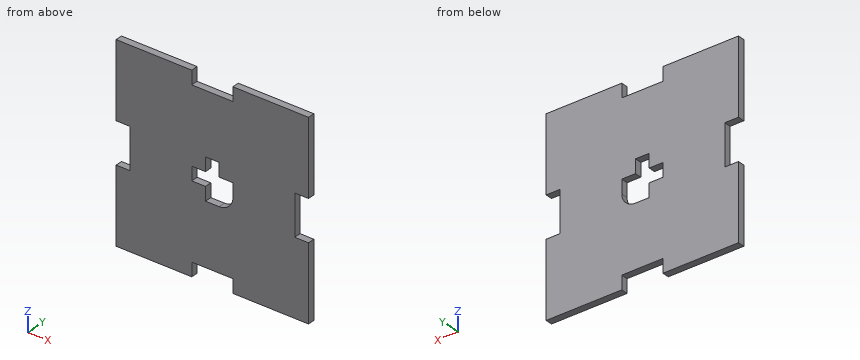
```python
from build123d import *

# Parameters (mm, degrees)
SKETCH1_W           = 88.9
SKETCH1_H           = 88.9
BOSS_EXTRUDE1_DEPTH = 3.175
CUT_EXTRUDE3_DEPTH  = 3.175
SKETCH4_W           = 19.05
SKETCH4_H           = 6.35
SKETCH4_W_2         = 6.35
SKETCH4_H_2         = 19.05
CUT_EXTRUDE2_DEPTH  = 3.175
SKETCH7_W           = 6.35
SKETCH7_H           = 6.35
CUT_EXTRUDE4_DEPTH  = 126.763669734
FILLET1_R           = 6.35


with BuildPart() as part:
    # Sketch1 → Boss-Extrude1 (new body)
    with BuildSketch(Plane(origin=(0, 0, 0), x_dir=(1, 0, 0), z_dir=(0, 1, 0))):
        with Locations((44.45, 44.45)):
            Rectangle(SKETCH1_W, SKETCH1_H)
    extrude(amount=BOSS_EXTRUDE1_DEPTH)

    # Sketch5 → Cut-Extrude3 (cut)
    with BuildSketch(Plane(origin=(0, 3.175, 0), x_dir=(1, 0, 0), z_dir=(0, 1, 0))):
        Polygon((41.275, 47.625), (41.275, 53.975), (47.625, 53.975), (47.625, 47.625), (53.975, 47.625), (53.975, 41.275), (47.625, 41.275), (47.625, 34.925), (41.275, 34.925), (41.275, 41.275), (34.925, 41.275), (34.925, 47.625), align=None)
    extrude(amount=-CUT_EXTRUDE3_DEPTH, mode=Mode.SUBTRACT)

    # Sketch4 → Cut-Extrude2 (cut)
    with BuildSketch(Plane(origin=(0, 3.175, 0), x_dir=(1, 0, 0), z_dir=(0, 1, 0))):
        with Locations((44.45, 85.725)):
            Rectangle(SKETCH4_W, SKETCH4_H)
        with Locations((85.725, 44.45)):
            Rectangle(SKETCH4_W_2, SKETCH4_H_2)
        with Locations((44.45, 3.175)):
            Rectangle(SKETCH4_W, SKETCH4_H)
        with Locations((3.175, 44.45)):
            Rectangle(SKETCH4_W_2, SKETCH4_H_2)
    extrude(amount=-CUT_EXTRUDE2_DEPTH, mode=Mode.SUBTRACT)

    # Sketch7 → Cut-Extrude4 (cut, through all)
    with BuildSketch(Plane(origin=(0, 3.175, 0), x_dir=(1, 0, 0), z_dir=(0, 1, 0))):
        with Locations((50.8, 50.8)):
            Rectangle(SKETCH7_W, SKETCH7_H)
    extrude(amount=-CUT_EXTRUDE4_DEPTH, mode=Mode.SUBTRACT)

    # Fillet1
    fillet1_edges = [part.edges().sort_by_distance(p)[0] for p in [
        (53.975, 1.5875, -53.975),
    ]]
    fillet(fillet1_edges, radius=FILLET1_R)


solid = part.part
```
Input: part model. Units: mm. Frame: model coordinates. Give positions to 0.01 mm unless a question says otherwise; leave off trailing zeros. Loops run counter-clockwise (first coordinate to the right, second up) from the corner with the lowest first, then second, coordinate; pieces in that order, holes last.
1) Section query B-B on x = 50. Return the cut outline in (y, z) (3 decimals).
A:
outline: (0, -82.55) - (3.175, -82.55) - (3.175, -53.514) - (0, -53.514) - close; (0, -41.275) - (3.175, -41.275) - (3.175, -6.35) - (0, -6.35) - close
2) Line query: L1, parallel to X at y = 0.7, z = -83 (3 decimals); L2, parallel to X at y = 0.55, z = -47.5 (3 decimals); L3, parallel to Z at x = 35.5, y = 0.4 (3 decimals). Output: solid intervals per line, ascending.
A:
L1: x = 0 to 34.925, 53.975 to 88.9
L2: x = 6.35 to 34.925, 53.975 to 82.55
L3: z = -82.55 to -47.625, -41.275 to -6.35
3) Contact query for flat-ended pins moving along their axis: pin 1 (1.6 mm diameter, centred on x = 47, y = 1, fed in from +Z); pin 2 (1.6 mm diameter, centred on y = 2, z = -45, fed in from -X); pin 3 (1 mm diameter, centred on x = 40, y = 1, fed in from -Z). Output: stop coordinate, or through.
A:
pin 1: stops at z = -6.35
pin 2: stops at x = 6.35
pin 3: stops at z = -82.55
